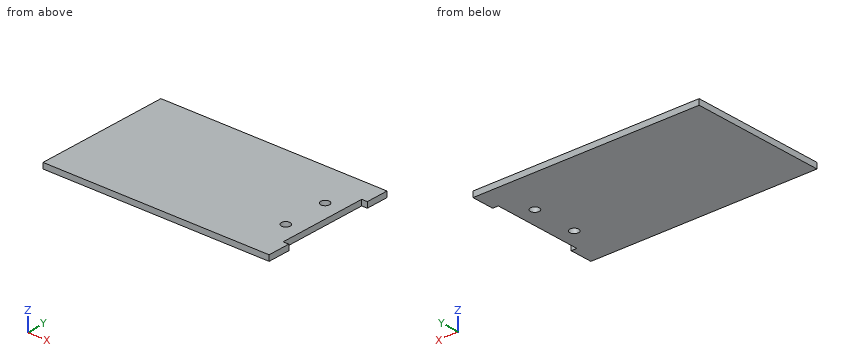
from build123d import *

# Parameters (mm, degrees)
SKETCH1_W                  = 76.2
SKETCH1_H                  = 127
BOSS_EXTRUDE1_DEPTH        = 3.175
F_9_0_196_DIAMETER_HOLE1_D = 4.9784
CUT_EXTRUDE1_DEPTH         = 75.121121315
CUT_EXTRUDE1_DEPTH_BACK    = 75.121121315


with BuildPart() as part:
    # Sketch1 → Boss-Extrude1 (new body)
    with BuildSketch(Plane(origin=(0, 0, 0), x_dir=(0, 1, 0), z_dir=(0, 0, 1))):
        Rectangle(SKETCH1_W, SKETCH1_H)
    extrude(amount=BOSS_EXTRUDE1_DEPTH)

    # #9 (0.196) Diameter Hole1 (through all)
    with Locations(Plane.XY.offset(3.175)):
        with Locations((50.8, -12.7), (50.8, 12.7)):
            Hole(F_9_0_196_DIAMETER_HOLE1_D / 2)

    # Sketch4 → Cut-Extrude1 (cut, two sides: drawn at the far end of the back side and taken through both)
    with BuildSketch(Plane.XY.offset(3.175).offset(-CUT_EXTRUDE1_DEPTH_BACK)):
        Polygon((357.480633142, 25.4), (63.5, 25.4), (60.325, 25.4), (60.325, -25.4), (63.5, -25.4), (357.480633142, -25.4), (945.441899427, -25.4), (945.441899427, 25.4), align=None)
    extrude(amount=CUT_EXTRUDE1_DEPTH + CUT_EXTRUDE1_DEPTH_BACK, mode=Mode.SUBTRACT)


solid = part.part
Input: part model. Units: mm. Frame: model coordinates. Give positions to 0.01 mm unless a question says otherwise; leave off trailing zeros. Order: outer loops, then holes, each group sorted by start corner. A loop starts at its lowest first (then second) coordinate and runs counter-clockwise, first axis right, second up. Notation, with made-up numbers: (69.5, -2) - (90.5, -2) arc R30 cw to (90.5, 25) - close; hole circle Ø3 at (16, -29). An arc over 180 degrees is marked (long way). Answer as a JSON object with one key per item and string values. Group by question number.
Q1. Cut plane A-A, the plane x = 50.8. Output: boundary loops of the cut face in (y, z) (3 decimals).
Q2. Cut plane C-C, the plane z = 2.4. Output: boundary loops of the cut face in (x, y) (3 decimals).
Q3. Cut plane B-B, the plane y = 12.7. Output: boundary loops of the cut face in (x, z) (3 decimals), then the cut area to 3 significant figures.
Q4. First-contact query: pin 1 Ø1 at (y, z) = (-11.5, 1.5) entering from +X (3 decimals). Flat tip, straight axial feed; report the tip coordinate or a pass-through.
Q5. Cut plane D-D, the plane y = -18. Output: boundary loops of the cut face in (x, z) (3 decimals).
Q6. Line query: probe 1 along Y at (x, z) = (50.8, 1.9); probe 2 along X at (y, z) = (13, 2.95) (3 decimals); probe 3 along X at (y, z) = (-23, 2.6) (3 decimals). Output: solid intervals per line, ascending.
Results:
{
 "1": {"outline": "(-38.1, 0) - (-15.189, 0) - (-15.189, 3.175) - (-38.1, 3.175) - close; (-10.211, 0) - (10.211, 0) - (10.211, 3.175) - (-10.211, 3.175) - close; (15.189, 0) - (38.1, 0) - (38.1, 3.175) - (15.189, 3.175) - close"},
 "2": {"outline": "(-63.5, -38.1) - (63.5, -38.1) - (63.5, -25.4) - (60.325, -25.4) - (60.325, 25.4) - (63.5, 25.4) - (63.5, 38.1) - (-63.5, 38.1) - close; hole circle Ø4.978 at (50.8, -12.7); hole circle Ø4.978 at (50.8, 12.7)"},
 "3": {"outline": "(-63.5, 0) - (48.311, 0) - (48.311, 3.175) - (-63.5, 3.175) - close; (53.289, 0) - (60.325, 0) - (60.325, 3.175) - (53.289, 3.175) - close", "area": "377 mm^2"},
 "4": {"pin 1": "x = 60.325"},
 "5": {"outline": "(-63.5, 0) - (60.325, 0) - (60.325, 3.175) - (-63.5, 3.175) - close"},
 "6": {"probe 1": "-38.1 to -15.19, -10.21 to 10.21, 15.19 to 38.1", "probe 2": "-63.5 to 48.329, 53.271 to 60.325", "probe 3": "-63.5 to 60.325"}
}
